The drawing under review shows one solid part. Ordinate dimensions are in mm from its lowest x, y, z. A direction names the side the tool comes from. Coordinates: 2 decimals unless noted, no trailing zeros. Order: outer loops, then holes, each group sorted by start corner. A loop starts at its lowest first (then second) coordinate and runs counter-clockwise, first axis right, second up. Notation, with made-up numbers: (-4.5, 35) - (46.5, 35) arc R30 ccw to (46.5, 73) - close; hole circle Ø6 at (-29.5, -36.75). An arc over 180 degrees is marked (long way). Write item = value, one per line. Start each with the question number.
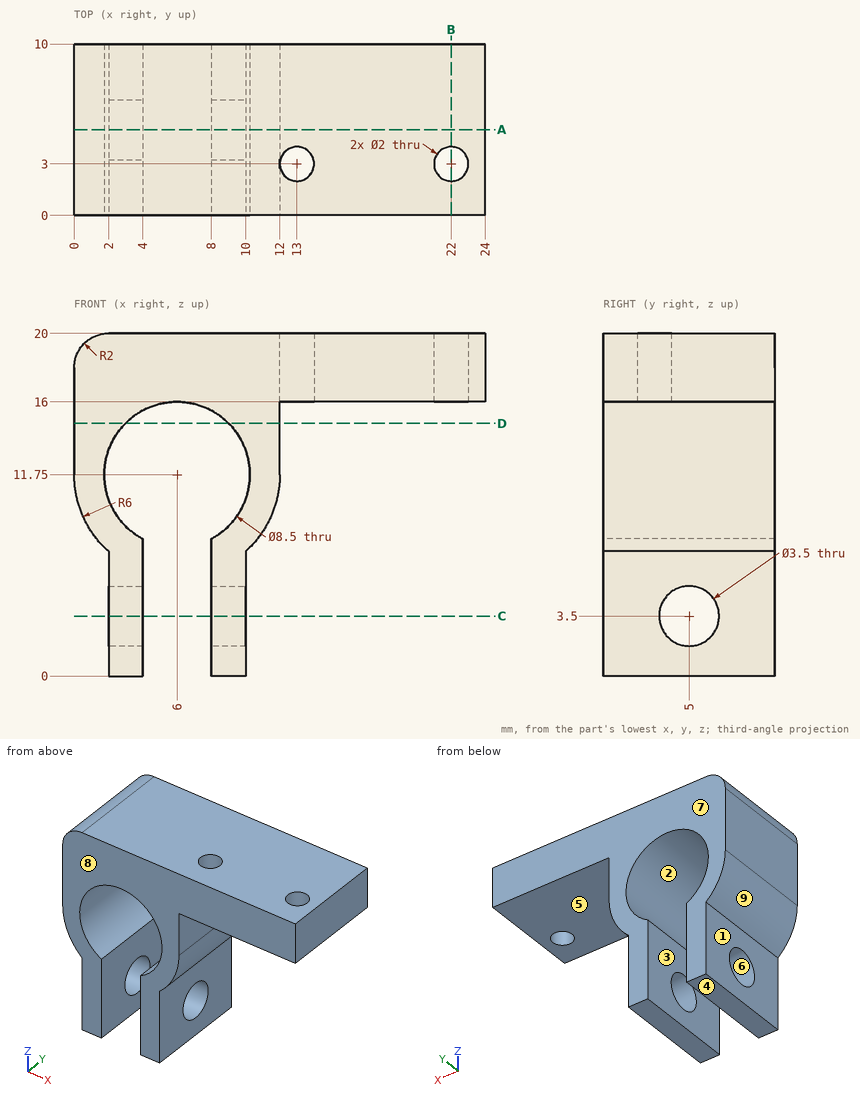
Item 1: For line 1 (Y direction, x = 2.8, z = 3.5); line 2 (X direction, y = 6, z = 11.5); line 3 (Z direction, x = 2.25, y = 6.5), list the stretches that pass through material, from the lowest coordinate up.
Item 2: Add section A-A on y = 5. Give the boundary of the cut face in (x, z), plus the area to 3 significant figures.
Item 3: Mouldability with a two-part tool opening along Y and no side actions: class the marked faces 6, 7, 8 and 9 as +Y half, -Y half, draft (parallel to the pull), parting line (faces both ways), or undercut.
Item 4: Add section B-B on x = 22. Give the boundary of the cut face in (y, z).
Item 5: For P1, Ø6, axis at x = 9, y = 6, coming from the -Z side; P2, Ø1.6, axis at x = 22, y = 3, coming from the +Z side; P3, Ø2, axis at y = 6.5, z = 3, coming from the +X side; P4, Ø1.3, axis at y = 5.5, z = 15, coming from the +X side, all flat-tipped, find the tip position at first contact; note any pin that passes through.
Item 6: Add section C-C on z = 3.5. Give the boundary of the cut face in (x, y), plus the area to 3 significant figures.
Item 7: For the marked faces 1, 2, 3, 4 and 5, list the 3-axis set-ups (+Z, -Z, +X, -X, +Y, -Y) from which the entire face can be reached by the end or side of a thin tool; tool diameter is ignored.
Item 8: Add section D-D on z = 14.75. Give the boundary of the cut face in (x, y).
Worked out:
q1.line_1 = 0 to 3.25, 6.75 to 10
q1.line_2 = 0.01 to 1.76, 10.24 to 11.99
q1.line_3 = 0 to 2.6, 4.4 to 9.75, 13.75 to 20
q2.outline = (0, 11.75) arc R6 ccw to (2, 7.28) - (2, 5.25) - (4, 5.25) - (4, 8) arc R4.25 cw (long way) to (8, 8) - (8, 5.25) - (10, 5.25) - (10, 7.28) arc R6 ccw to (12, 11.75) - (12, 16) - (24, 16) - (24, 20) - (2, 20) arc R2 ccw to (0, 18) - close; (2, 0) - (4, 0) - (4, 1.75) - (2, 1.75) - close; (8, 0) - (10, 0) - (10, 1.75) - (8, 1.75) - close
q2.area = 151 mm2
q3.face_6 = undercut
q3.face_7 = +Y half
q3.face_8 = -Y half
q3.face_9 = draft
q4.outline = (0, 16) - (2, 16) - (2, 20) - (0, 20) - close; (4, 16) - (10, 16) - (10, 20) - (4, 20) - close
q5.P1 = 0
q5.P2 = through
q5.P3 = 10
q5.P4 = 12
q6.outline = (2, 0) - (4, 0) - (4, 3.25) - (2, 3.25) - close; (2, 6.75) - (4, 6.75) - (4, 10) - (2, 10) - close; (8, 0) - (10, 0) - (10, 3.25) - (8, 3.25) - close; (8, 6.75) - (10, 6.75) - (10, 10) - (8, 10) - close
q6.area = 26.0 mm2
q7.face_1 = -Z, -X, +Y, -Y
q7.face_2 = +Y, -Y
q7.face_3 = -Z, +Y, -Y
q7.face_4 = -Z, +X, -X, +Y, -Y
q7.face_5 = -Z, +X, +Y, -Y
q8.outline = (0, 0) - (2.99, 0) - (2.99, 10) - (0, 10) - close; (9.01, 0) - (12, 0) - (12, 10) - (9.01, 10) - close
